Read the model definition and answer for the solid it produces. Units are mm, in the model's axes. Coordinates: 2 decimals unless noted, no trailing zeros. Loops run counter-clockwise (first coordinate to the right, second up) from the corner with the lowest first, then second, coordinate; pieces in that order, holes last. Notation, with made-up numbers: (62.5, 4) - (81.5, 4) arc R28 ccw to (81.5, 34) - close; hole circle Ø3 at (51, -24). An arc over 180 degrees is marked (long way). One line per item, written item: value. Start each with the question number.
from build123d import *

# Parameters (mm, degrees)
SKETCH1_W                      = 469.9
SKETCH1_H                      = 2413
SKETCH1_R                      = 203.2
BOSS_EXTRUDE1_DEPTH            = 6.35
F_1_4_CLEARANCE_HOLE1_D        = 6.7564
F_5_16_0_3125_DIAMETER_HOLE1_D = 7.9375


with BuildPart() as part:
    # Sketch1 → Boss-Extrude1 (new body)
    with BuildSketch(Plane.XY):
        with Locations((0, 1206.5)):
            Rectangle(SKETCH1_W, SKETCH1_H)
        with Locations((0, 695.96)):
            Circle(SKETCH1_R, mode=Mode.SUBTRACT)
        with Locations((0, 1407.16)):
            Circle(SKETCH1_R, mode=Mode.SUBTRACT)
        with Locations((0, 2118.36)):
            Circle(SKETCH1_R, mode=Mode.SUBTRACT)
    extrude(amount=BOSS_EXTRUDE1_DEPTH)

    # 1/4 Clearance Hole1 (through all)
    with Locations(Plane.XY.offset(6.35)):
        with Locations((44.571271172, 378.545152647), (118.174819136, 358.82314141), (-44.571271172, 378.545152647), (-118.174819136, 358.82314141), (44.571271172, 1089.745152647), (118.174819136, 1070.02314141), (-44.571271172, 1089.745152647), (-118.174819136, 1070.02314141), (44.571271172, 1800.945152647), (118.174819136, 1781.22314141), (-44.571271172, 1800.945152647), (-118.174819136, 1781.22314141), (189.372114723, 379.189906028), (-189.372114723, 379.189906028), (-189.372114723, 1090.389906028), (-189.372114723, 1801.589906028), (189.372114723, 1801.589906028), (189.372114723, 1090.389906028)):
            Hole(F_1_4_CLEARANCE_HOLE1_D / 2)

    # 5/16 (0.3125) Diameter Hole1 (through all)
    with Locations(Plane.XY.offset(6.35)):
        with Locations((-114.3, 254.635), (-114.3, 210.185), (-196.85, 177.8), (196.85, 177.8), (114.3, 210.185), (114.3, 254.635), (-114.3, 965.835), (-114.3, 921.385), (-196.85, 889), (196.85, 889), (114.3, 921.385), (114.3, 965.835), (-114.3, 1677.035), (-114.3, 1632.585), (-196.85, 1600.2), (196.85, 1600.2), (114.3, 1632.585), (114.3, 1677.035), (-114.3, 2388.235), (-114.3, 2343.785), (-196.85, 2311.4), (196.85, 2311.4), (114.3, 2343.785), (114.3, 2388.235)):
            Hole(F_5_16_0_3125_DIAMETER_HOLE1_D / 2)


solid = part.part
1) Section D-D, the plane z = 3 is taken. State how many separate pieces and enclosed holes the cut face has, and give its area (3 significant figures).
2) Section A-A, the plane y = 695.96 is taken. Determine the outline of the cut face in (x, z).
3) Section B-B, the plane x = 0 is taken. Determine the outline of the cut face in (y, z).
4) Straight lines are drawn through the part: L1, parallel to X at y = 1069, z = 5.75; L2, parallel to Y at x = -137.5, z = 3.5; L3, parallel to Y at x = -35.5, z = 2.25. For each, find the intervals that lie inside material, in ascending order.
5) Determine the mould class of faces 1 (the cylindrical face through (109.24, 2289.7, 3.13)), 2 (the flat face through (-3, 955, 0)), 3 (the cylindrical face through (-44.05, 1208.792, 3.131)) for opening direction X: released by +X, released by -X, zero draft, split by the parting line, or undercut.
6) Section C-C, the plane x = 159 is taken. Determine the outline of the cut face in (y, z).
Answer below:
1. separate pieces: 1
1. enclosed holes: 45
1. area: 743,000 mm2
2. outline: (-234.95, 0) - (-203.2, 0) - (-203.2, 6.35) - (-234.95, 6.35) - close; (203.2, 0) - (234.95, 0) - (234.95, 6.35) - (203.2, 6.35) - close
3. outline: (0, 0) - (492.76, 0) - (492.76, 6.35) - (0, 6.35) - close; (899.16, 0) - (1203.96, 0) - (1203.96, 6.35) - (899.16, 6.35) - close; (1610.36, 0) - (1915.16, 0) - (1915.16, 6.35) - (1610.36, 6.35) - close; (2321.56, 0) - (2413, 0) - (2413, 6.35) - (2321.56, 6.35) - close
4. L1: -234.95 to -121.39, -114.96 to 114.96, 121.39 to 234.95
4. L2: 0 to 546.35, 845.57 to 1257.55, 1556.77 to 1968.75, 2267.97 to 2413
4. L3: 0 to 495.89, 896.03 to 1207.09, 1607.23 to 1918.29, 2318.43 to 2413
5. face 1: undercut
5. face 2: zero draft
5. face 3: undercut
6. outline: (0, 0) - (569.43, 0) - (569.43, 6.35) - (0, 6.35) - close; (822.49, 0) - (1280.63, 0) - (1280.63, 6.35) - (822.49, 6.35) - close; (1533.69, 0) - (1991.83, 0) - (1991.83, 6.35) - (1533.69, 6.35) - close; (2244.89, 0) - (2413, 0) - (2413, 6.35) - (2244.89, 6.35) - close
